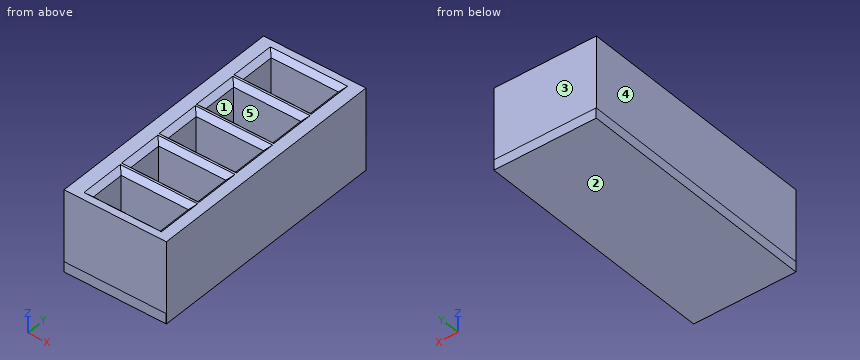
```python
from build123d import *

# Parameters (mm, degrees)
F0_W     = 31.75
F0_H     = 76.2
F0_W_2   = 20.828
F0_H_2   = 10.668
F1_DEPTH = 25.4
F2_W     = 31.691335
F2_H     = 76.259181
F3_DEPTH = 3.175
F4_SIZE  = 1.5875


with BuildPart() as f1:
    # F0 (on Top) → F1 (new body)
    with BuildSketch(Plane.XY):
        with Locations((15.875, 38.1)):
            Rectangle(F0_W, F0_H)
        with Locations((16.382345, 9.146222)):
            Rectangle(F0_W_2, F0_H_2, mode=Mode.SUBTRACT)
        with Locations((16.255509, 23.623667)):
            Rectangle(F0_W_2, F0_H_2, mode=Mode.SUBTRACT)
        with Locations((16.128672, 38.101111)):
            Rectangle(F0_W_2, F0_H_2, mode=Mode.SUBTRACT)
        with Locations((16.001836, 52.578556)):
            Rectangle(F0_W_2, F0_H_2, mode=Mode.SUBTRACT)
        with Locations((15.875, 67.056)):
            Rectangle(F0_W_2, F0_H_2, mode=Mode.SUBTRACT)
    extrude(amount=F1_DEPTH)

    # F2 (on Top) → F3 (join)
    with BuildSketch(Plane.XY):
        with Locations((15.845667, 38.12959)):
            Rectangle(F2_W, F2_H)
    extrude(amount=F3_DEPTH)

    # F4
    f4_edges = [f1.edges().sort_by_distance(p)[0] for p in [
        (5.968345, 9.146222, 25.4),
        (16.382345, 3.812222, 25.4),
        (26.796345, 9.146222, 25.4),
        (16.382345, 14.480222, 25.4),
        (16.255509, 18.289667, 25.4),
        (5.841509, 23.623667, 25.4),
        (26.669509, 23.623667, 25.4),
        (16.255509, 28.957667, 25.4),
        (16.128672, 32.767111, 25.4),
        (5.714672, 38.101111, 25.4),
        (26.542672, 38.101111, 25.4),
        (16.128672, 43.435111, 25.4),
        (16.001836, 57.912556, 25.4),
        (5.587836, 52.578556, 25.4),
        (16.001836, 47.244556, 25.4),
        (26.415836, 52.578556, 25.4),
        (15.875, 61.722, 25.4),
        (5.461, 67.056, 25.4),
        (15.875, 72.39, 25.4),
        (26.289, 67.056, 25.4),
    ]]
    chamfer(f4_edges, length=F4_SIZE)


solid = f1.part
```
The listing builds one solid part. Answer for the finished solid, in the listing's coordinates (mm). Face numbers are marked on the shaded views. A direction names the side the tool comes from. Give positions to 0.01 mm unless a question says otherwise; leave off trailing zeros. Write each loop counter-clockwise with the first axis right and the second up, starting at its lowest first coordinate (ties: lowest second). Pieces come first, ordered by that corner, then holes. Notation, with made-up numbers: M 70,61 L 128,61 A21 cw 128,82 Z; hole C -2,76 d11. An arc over 180 degrees is marked long. Write each question's results on one line, items separated by ' | '.
Q1. Section A-A, the plane z = 17.5 is taken. Write down the section's boundary in (x, y).
Output values:
outline: M 0,0 L 31.75,0 L 31.75,76.2 L 0,76.2 Z; hole M 5.46,61.72 L 26.29,61.72 L 26.29,72.39 L 5.46,72.39 Z; hole M 5.59,47.24 L 26.42,47.24 L 26.42,57.91 L 5.59,57.91 Z; hole M 5.71,32.77 L 26.54,32.77 L 26.54,43.44 L 5.71,43.44 Z; hole M 5.84,18.29 L 26.67,18.29 L 26.67,28.96 L 5.84,28.96 Z; hole M 5.97,3.81 L 26.8,3.81 L 26.8,14.48 L 5.97,14.48 Z
Q2. For a pull along X with two mould halves and no side action, classify the marked faces 3, 4 and 5 as released by +X, released by -X, zero draft, split by the parting line, or undercut.
Output values:
face 3: zero draft | face 4: released by -X | face 5: undercut
Q3. Flat-ended cylindrical pins translate along their axes: P1, Ø11.5, axis at x = 18, y = 51.5, coming from the +Z side; P2, Ø10.5, axis at x = 14, z = 17.5, coming from the +Y side. Find the tip coordinate at first contact, or state that the pin passes through.
Output values:
P1: z = 25.31 | P2: y = 76.2
Q4. Consider L1, parallel to Y at x = 16, z = 13.5; L2, parallel to X at y = 9.5, z = 5; L3, parallel to X at y = 28, z = 6.5. Determine where each line is inside the solid, lowest interval first. Write a range as from..to.
Output values:
L1: 0..3.81, 14.48..18.29, 28.96..32.77, 43.44..47.24, 57.91..61.72, 72.39..76.2 | L2: 0..5.97, 26.8..31.75 | L3: 0..5.84, 26.67..31.75
Q5. A tool of negligible diameter and unlimited length cuts with its end or side. For the marked faces 1 and 2, from which of +Z, -Z, +X, -X, +Y, -Y can it reach the whole face along a straight path? Write none if from no direction.
Output values:
face 1: +Z | face 2: -Z, +X, -X, +Y, -Y
